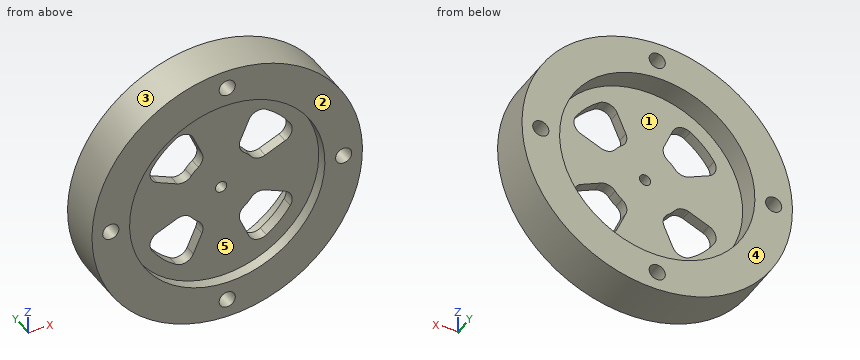
from build123d import *

# Parameters (mm, degrees)
CUT_EXTRUDE1_REACH               = 53.264
F_18_0_1695_DIAMETER_HOLE1_D     = 4.3053
F_18_0_1695_DIAMETER_HOLE1_DEPTH = 381
F_18_0_1695_DIAMETER_HOLE1_TIP   = 1.293442612
CUT_EXTRUDE2_REACH               = 53.264
SKETCH5_R                        = 1.5


with BuildPart() as part:
    # Sketch1 → Revolve1 (revolve)
    with BuildSketch(Plane.XY, mode=Mode.PRIVATE) as revolve1_sk:
        Polygon((0, 3), (26, 3), (26, 0), (36, 0), (36, 12), (26, 12), (26, 6), (0, 6), align=None)
    revolve(revolve1_sk.sketch.rotate(Axis((0, 0, 0), (0, 1, 0)), 90), axis=Axis((0, 0, 0), (0, 1, 0)))

    # Sketch2 → Cut-Extrude1 (cut, up to next)
    with BuildSketch(Plane(origin=(0, 6, 0), x_dir=(1, 0, 0), z_dir=(0, 1, 0)), mode=Mode.PRIVATE) as cut_extrude1_sk1:
        with BuildLine():
            Line((7.398917645, 17.016345603), (5.098689446, 11.726182923))
            ThreePointArc((5.098689446, 11.726182923), (4.936869827, 9.663717077), (6.079965983, 7.939396303))
            ThreePointArc((6.079965983, 7.939396303), (7.071067812, 7.071067812), (7.939396303, 6.079965983))
            ThreePointArc((7.939396303, 6.079965983), (9.663717077, 4.936869827), (11.726182923, 5.098689446))
            Line((11.726182923, 5.098689446), (17.016345603, 7.398917645))
            ThreePointArc((17.016345603, 7.398917645), (18.792276888, 9.401129193), (18.406745328, 12.049552955))
            ThreePointArc((18.406745328, 12.049552955), (15.556349186, 15.556349186), (12.049552955, 18.406745328))
            ThreePointArc((12.049552955, 18.406745328), (9.401129193, 18.792276888), (7.398917645, 17.016345603))
        make_face()
    cut_extrude1_tool1 = extrude(cut_extrude1_sk1.sketch, amount=-CUT_EXTRUDE1_REACH, mode=Mode.PRIVATE) & part.part
    # Sketch2 → Cut-Extrude1 (cut, up to next)
    with BuildSketch(Plane(origin=(0, 6, 0), x_dir=(1, 0, 0), z_dir=(0, 1, 0)), mode=Mode.PRIVATE) as cut_extrude1_sk2:
        with BuildLine():
            Line((-7.398917645, 17.016345603), (-5.098689446, 11.726182923))
            ThreePointArc((-5.098689446, 11.726182923), (-4.936869827, 9.663717077), (-6.079965983, 7.939396303))
            ThreePointArc((-6.079965983, 7.939396303), (-7.071067812, 7.071067812), (-7.939396303, 6.079965983))
            ThreePointArc((-7.939396303, 6.079965983), (-9.663717077, 4.936869827), (-11.726182923, 5.098689446))
            Line((-11.726182923, 5.098689446), (-17.016345603, 7.398917645))
            ThreePointArc((-17.016345603, 7.398917645), (-18.792276888, 9.401129193), (-18.406745328, 12.049552955))
            ThreePointArc((-18.406745328, 12.049552955), (-15.556349186, 15.556349186), (-12.049552955, 18.406745328))
            ThreePointArc((-12.049552955, 18.406745328), (-9.401129193, 18.792276888), (-7.398917645, 17.016345603))
        make_face()
    cut_extrude1_tool2 = extrude(cut_extrude1_sk2.sketch, amount=-CUT_EXTRUDE1_REACH, mode=Mode.PRIVATE) & part.part
    # Sketch2 → Cut-Extrude1 (cut, up to next)
    with BuildSketch(Plane(origin=(0, 6, 0), x_dir=(1, 0, 0), z_dir=(0, 1, 0)), mode=Mode.PRIVATE) as cut_extrude1_sk3:
        with BuildLine():
            Line((17.016345603, -7.398917645), (11.726182923, -5.098689446))
            ThreePointArc((11.726182923, -5.098689446), (9.663717077, -4.936869827), (7.939396303, -6.079965983))
            ThreePointArc((7.939396303, -6.079965983), (7.071067812, -7.071067812), (6.079965983, -7.939396303))
            ThreePointArc((6.079965983, -7.939396303), (4.936869827, -9.663717077), (5.098689446, -11.726182923))
            Line((5.098689446, -11.726182923), (7.398917645, -17.016345603))
            ThreePointArc((7.398917645, -17.016345603), (9.401129193, -18.792276888), (12.049552955, -18.406745328))
            ThreePointArc((12.049552955, -18.406745328), (15.556349186, -15.556349186), (18.406745328, -12.049552955))
            ThreePointArc((18.406745328, -12.049552955), (18.792276888, -9.401129193), (17.016345603, -7.398917645))
        make_face()
    cut_extrude1_tool3 = extrude(cut_extrude1_sk3.sketch, amount=-CUT_EXTRUDE1_REACH, mode=Mode.PRIVATE) & part.part
    # Sketch2 → Cut-Extrude1 (cut, up to next)
    with BuildSketch(Plane(origin=(0, 6, 0), x_dir=(1, 0, 0), z_dir=(0, 1, 0)), mode=Mode.PRIVATE) as cut_extrude1_sk4:
        with BuildLine():
            Line((-7.398917645, -17.016345603), (-5.098689446, -11.726182923))
            ThreePointArc((-5.098689446, -11.726182923), (-4.936869827, -9.663717077), (-6.079965983, -7.939396303))
            ThreePointArc((-6.079965983, -7.939396303), (-7.071067812, -7.071067812), (-7.939396303, -6.079965983))
            ThreePointArc((-7.939396303, -6.079965983), (-9.663717077, -4.936869827), (-11.726182923, -5.098689446))
            Line((-11.726182923, -5.098689446), (-17.016345603, -7.398917645))
            ThreePointArc((-17.016345603, -7.398917645), (-18.792276888, -9.401129193), (-18.406745328, -12.049552955))
            ThreePointArc((-18.406745328, -12.049552955), (-15.556349186, -15.556349186), (-12.049552955, -18.406745328))
            ThreePointArc((-12.049552955, -18.406745328), (-9.401129193, -18.792276888), (-7.398917645, -17.016345603))
        make_face()
    cut_extrude1_tool4 = extrude(cut_extrude1_sk4.sketch, amount=-CUT_EXTRUDE1_REACH, mode=Mode.PRIVATE) & part.part
    add(cut_extrude1_tool1.solids().sort_by_distance((11.555905, 6, -11.555905))[0], mode=Mode.SUBTRACT)
    add(cut_extrude1_tool2.solids().sort_by_distance((-11.555905, 6, -11.555905))[0], mode=Mode.SUBTRACT)
    add(cut_extrude1_tool3.solids().sort_by_distance((11.555905, 6, 11.555905))[0], mode=Mode.SUBTRACT)
    add(cut_extrude1_tool4.solids().sort_by_distance((-11.555905, 6, 11.555905))[0], mode=Mode.SUBTRACT)

    # 18 _0.1695_ Diameter Hole1
    with Locations(Plane(origin=(0, 12, 0), x_dir=(1, 0, 0), z_dir=(0, 1, 0))):
        with Locations((0, 31), (0, -31), (-31, 0), (31, 0)):
            Hole(F_18_0_1695_DIAMETER_HOLE1_D / 2, depth=F_18_0_1695_DIAMETER_HOLE1_DEPTH)
            with Locations((0, 0, -(F_18_0_1695_DIAMETER_HOLE1_DEPTH + F_18_0_1695_DIAMETER_HOLE1_TIP / 2))):  # 118° drill point
                Cone(0, F_18_0_1695_DIAMETER_HOLE1_D / 2, F_18_0_1695_DIAMETER_HOLE1_TIP, mode=Mode.SUBTRACT)

    # Sketch5 → Cut-Extrude2 (cut, up to next)
    with BuildSketch(Plane(origin=(0, 6, 0), x_dir=(1, 0, 0), z_dir=(0, 1, 0)), mode=Mode.PRIVATE) as cut_extrude2_sk1:
        with Locations(Location((0, 0, 0), (0, 0, 270))):
            Circle(SKETCH5_R)
    cut_extrude2_tool1 = extrude(cut_extrude2_sk1.sketch, amount=-CUT_EXTRUDE2_REACH, mode=Mode.PRIVATE) & part.part
    add(cut_extrude2_tool1.solids().sort_by_distance((0, 6, 0))[0], mode=Mode.SUBTRACT)


solid = part.part
Part model, mm, in its own coordinate system. Face numbers are marked on the shaded views. A direction names the side the tool comes from. Give positions to 0.01 mm unless a question says otherwise; leave off trailing zeros. Loops run counter-clockwise (first coordinate to the right, second up) from the corner with the lowest first, then second, coordinate; pieces in that order, holes last. Notation, with made-up numbers: M 80.25,64.5 L 111.25,64.5 A25 cw 111.25,77.5 Z; hole C 67,-36 d2. An arc over 180 degrees is marked long. Put each result on its own line as item: value. Start each with the question number.
1) Saw through at A-A (x = 0). List the corners of the cut face in (y, z).
2) Saw through at D-D (y = 11). List the corners of the cut face in (x, z).
3) 3-axis set-ups, long thin cutter, end or side, ignore diameter. For the marked faces 1 and 2: which of +Z, -Z, +X, -X, +Y, -Y reach the whole face in a straight line?
4) Probe probe 1 along Z at (x, y) = (1, 9.5); probe 2 along X at (y, z) = (4.5, 7); probe 3 along X at (y, z) = (9.75, 31). List the from-to ranges inside material, lowest first.
5) Pull direction Z, two halves, no side cores. Call the marked faces 3, 4 and 5: +Z half, -Z half, draft (parallel to the pull), parting line (faces both ways), or undercut.
6) Saw through at B-B (z = 0). List the corners of the cut face in (x, y).
7) Flat gauge pins, fed straight in: pin 1 (3.5 mm diameter, centred on x = 0, z = 0, fed in from +Y); pin 2 (1 mm diameter, centred on x = -4.5, y = 4.5, fed in from +Z); pin 3 (4 mm diameter, centred on y = 2.5, z = -22, fed in from +X). Where does each tip first touch, or does it go through?
8) Saw through at C-C (z = 31). List the corners of the cut face in (x, y), then the cut area to 3 significant figures.
Numbers:
1. outline: M 0,-36 L 12,-36 L 12,-33.15 L 0,-33.15 Z; M 0,-28.85 L 12,-28.85 L 12,-26 L 6,-26 L 6,-1.5 L 3,-1.5 L 3,-26 L 0,-26 Z; M 0,26 L 3,26 L 3,1.5 L 6,1.5 L 6,26 L 12,26 L 12,28.85 L 0,28.85 Z; M 0,33.15 L 12,33.15 L 12,36 L 0,36 Z
2. outline: C 0,0 d72; hole C -31,0 d4.31; hole C 0,0 d52; hole C 0,-31 d4.31; hole C 0,31 d4.31; hole C 31,0 d4.31
3. face 1: +Y
3. face 2: +Z, -Z, +X, -X, -Y
4. probe 1: -35.99 to -32.91, -29.09 to -25.98, 25.98 to 29.09, 32.91 to 35.99
4. probe 2: -35.31 to -16.1, -7.14 to 7.14, 16.1 to 35.31
4. probe 3: -18.3 to -2.15, 2.15 to 18.3
5. face 3: parting line
5. face 4: draft
5. face 5: undercut
6. outline: M -36,0 L -33.15,0 L -33.15,12 L -36,12 Z; M -28.85,0 L -26,0 L -26,3 L -1.5,3 L -1.5,6 L -26,6 L -26,12 L -28.85,12 Z; M 1.5,3 L 26,3 L 26,0 L 28.85,0 L 28.85,12 L 26,12 L 26,6 L 1.5,6 Z; M 33.15,0 L 36,0 L 36,12 L 33.15,12 Z
7. pin 1: y = 6
7. pin 2: z = 35.78
7. pin 3: x = 29.93
8. outline: M -18.3,0 L -2.15,0 L -2.15,12 L -18.3,12 Z; M 2.15,0 L 18.3,0 L 18.3,12 L 2.15,12 Z
8. area: 388 mm^2
